```python
from build123d import *

# Parameters (mm, degrees)
SKETCH_3_W            = 95.96
SKETCH_3_H            = 56.19
EXTRUDE_2_DEPTH       = 2
SKETCH_4_W            = 97.56
SKETCH_4_H            = 57.79
SKETCH_4_W_2          = 95.96
SKETCH_4_H_2          = 56.19
CUT_EXTRUDE_1_DEPTH   = 2
SKETCH_5_R            = 3.6
SKETCH_5_R_2          = 2.4
EXTRUDE_1_DEPTH       = 4.6
EXTRUDE_START         = -2
EXTRUDE_3_DEPTH       = 2
CHAMFER_1_SIZE        = 1.8
SKETCH_8_W            = 10
SKETCH_8_H            = 75.2
EXTRUDE_3_2_DEPTH     = 2
FILLET_1_R            = 4
SKETCH_9_R            = 5.5
CUT_EXTRUDE_1_2_DEPTH = 2
SKETCH_11_R           = 2.4
SKETCH_11_R_2         = 1
EXTRUDE_4_DEPTH       = 4.6
SKETCH_14_W           = 10
SKETCH_14_H           = 1
EXTRUDE_4_2_DEPTH     = 3
CHAMFER_2_SIZE        = 3
CHAMFER_3_SIZE        = 3


with BuildPart() as part:
    # Эскиз3 → Бобышка-Вытянуть2 (new body)
    with BuildSketch(Plane.XY):
        with BuildLine():
            Line((-57.5, -37), (57.5, -37))
            ThreePointArc((57.5, -37), (59.267766953, -36.267766953), (60, -34.5))
            Line((60, -34.5), (60, 34.5))
            ThreePointArc((60, 34.5), (59.267766953, 36.267766953), (57.5, 37))
            Line((57.5, 37), (-57.5, 37))
            ThreePointArc((-57.5, 37), (-59.267766953, 36.267766953), (-60, 34.5))
            Line((-60, 34.5), (-60, -34.5))
            ThreePointArc((-60, -34.5), (-59.267766953, -36.267766953), (-57.5, -37))
        make_face()
        with Locations((0, 2.375)):
            Rectangle(SKETCH_3_W, SKETCH_3_H, mode=Mode.SUBTRACT)
    extrude(amount=EXTRUDE_2_DEPTH)

    # Эскиз4 → Cut-Extrude 1 (cut)
    with BuildSketch(Plane.XY.offset(2)):
        with Locations((0, 2.375)):
            Rectangle(SKETCH_4_W, SKETCH_4_H)
        with Locations((0, 2.375)):
            Rectangle(SKETCH_4_W_2, SKETCH_4_H_2, mode=Mode.SUBTRACT)
    extrude(amount=-CUT_EXTRUDE_1_DEPTH, mode=Mode.SUBTRACT)

    # Эскиз5 → Вытянуть-Тонкостенный1 (add)
    # profile 1 of 4: a face of its own
    with BuildSketch(Plane(origin=(0, 0, 0), x_dir=(-1, 0, 0), z_dir=(0, 0, -1))):
        with Locations((56.75, 33.75)):
            Circle(SKETCH_5_R)
        with Locations((56.75, 33.75)):
            Circle(SKETCH_5_R_2, mode=Mode.SUBTRACT)
    # profile 2 of 4: a face of its own
    with BuildSketch(Plane(origin=(0, 0, 0), x_dir=(-1, 0, 0), z_dir=(0, 0, -1))):
        with Locations((-56.75, 33.75)):
            Circle(SKETCH_5_R)
        with Locations((-56.75, 33.75)):
            Circle(SKETCH_5_R_2, mode=Mode.SUBTRACT)
    # profile 3 of 4: a face of its own
    with BuildSketch(Plane(origin=(0, 0, 0), x_dir=(-1, 0, 0), z_dir=(0, 0, -1))):
        with Locations((-56.75, -33.75)):
            Circle(SKETCH_5_R)
        with Locations((-56.75, -33.75)):
            Circle(SKETCH_5_R_2, mode=Mode.SUBTRACT)
    # profile 4 of 4: a face of its own
    with BuildSketch(Plane(origin=(0, 0, 0), x_dir=(-1, 0, 0), z_dir=(0, 0, -1))):
        with Locations((56.75, -33.75)):
            Circle(SKETCH_5_R)
        with Locations((56.75, -33.75)):
            Circle(SKETCH_5_R_2, mode=Mode.SUBTRACT)
    extrude(amount=EXTRUDE_1_DEPTH)

    # Эскиз7 → Extrude 3 (add)
    with BuildSketch(Plane.XY.offset(2).offset(EXTRUDE_START)):
        with BuildLine():
            Line((-60.6, 34.5), (-60.6, -34.5))
            ThreePointArc((-60.6, -34.5), (-59.692031022, -36.692031022), (-57.5, -37.6))
            Line((-57.5, -37.6), (57.5, -37.6))
            ThreePointArc((57.5, -37.6), (59.692031022, -36.692031022), (60.6, -34.5))
            Line((60.6, -34.5), (60.6, 34.5))
            ThreePointArc((60.6, 34.5), (59.692031022, 36.692031022), (57.5, 37.6))
            Line((57.5, 37.6), (-57.5, 37.6))
            ThreePointArc((-57.5, 37.6), (-59.692031022, 36.692031022), (-60.6, 34.5))
        make_face()
        with BuildLine():
            Line((-60, 34.5), (-60, -34.5))
            ThreePointArc((-60, -34.5), (-59.267766953, -36.267766953), (-57.5, -37))
            Line((-57.5, -37), (57.5, -37))
            ThreePointArc((57.5, -37), (59.267766953, -36.267766953), (60, -34.5))
            Line((60, -34.5), (60, 34.5))
            ThreePointArc((60, 34.5), (59.267766953, 36.267766953), (57.5, 37))
            Line((57.5, 37), (-57.5, 37))
            ThreePointArc((-57.5, 37), (-59.267766953, 36.267766953), (-60, 34.5))
        make_face(mode=Mode.SUBTRACT)
    extrude(amount=EXTRUDE_3_DEPTH)

    # Фаска1
    chamfer_1_edges = [part.edges().sort_by_distance(p)[0] for p in [
        (0, 31.27, 2),
        (-48.78, 2.375, 2),
        (0, -26.52, 2),
        (48.78, 2.375, 2),
    ]]
    chamfer(chamfer_1_edges, length=CHAMFER_1_SIZE)

    # Эскиз8 → Extrude 3 2 (add)
    with BuildSketch(Plane.XY.offset(2)):
        with Locations((62.5, 0)):
            Rectangle(SKETCH_8_W, SKETCH_8_H)
        with Locations((-62.5, 0)):
            Rectangle(SKETCH_8_W, SKETCH_8_H)
    extrude(amount=-EXTRUDE_3_2_DEPTH)

    # Скругление1
    fillet_1_edges = [part.edges().sort_by_distance(p)[0] for p in [
        (67.5, 37.6, 1),
        (67.5, -37.6, 1),
        (-67.5, -37.6, 1),
        (-67.5, 37.6, 1),
    ]]
    fillet(fillet_1_edges, radius=FILLET_1_R)

    # Эскиз9 → Cut-Extrude 1 2 (cut)
    with BuildSketch(Plane.XY.offset(2)):
        with Locations((59.1, 9.48)):
            Circle(SKETCH_9_R)
        with Locations((59.1, -6.52)):
            Circle(SKETCH_9_R)
    extrude(amount=-CUT_EXTRUDE_1_2_DEPTH, mode=Mode.SUBTRACT)

    # Эскиз11 → Extrude 4 (add)
    # profile 1 of 4: a face of its own
    with BuildSketch(Plane(origin=(0, 0, 0), x_dir=(-1, 0, 0), z_dir=(0, 0, -1))):
        with Locations((-56.75, 33.75)):
            Circle(SKETCH_11_R)
        with Locations((-56.75, 33.75)):
            Circle(SKETCH_11_R_2, mode=Mode.SUBTRACT)
    # profile 2 of 4: a face of its own
    with BuildSketch(Plane(origin=(0, 0, 0), x_dir=(-1, 0, 0), z_dir=(0, 0, -1))):
        with Locations((56.75, 33.75)):
            Circle(SKETCH_11_R)
        with Locations((56.75, 33.75)):
            Circle(SKETCH_11_R_2, mode=Mode.SUBTRACT)
    # profile 3 of 4: a face of its own
    with BuildSketch(Plane(origin=(0, 0, 0), x_dir=(-1, 0, 0), z_dir=(0, 0, -1))):
        with Locations((56.75, -33.75)):
            Circle(SKETCH_11_R)
        with Locations((56.75, -33.75)):
            Circle(SKETCH_11_R_2, mode=Mode.SUBTRACT)
    # profile 4 of 4: a face of its own
    with BuildSketch(Plane(origin=(0, 0, 0), x_dir=(-1, 0, 0), z_dir=(0, 0, -1))):
        with Locations((-56.75, -33.75)):
            Circle(SKETCH_11_R)
        with Locations((-56.75, -33.75)):
            Circle(SKETCH_11_R_2, mode=Mode.SUBTRACT)
    extrude(amount=EXTRUDE_4_DEPTH)

    # Эскиз14 → Extrude 4 2 (add)
    with BuildSketch(Plane(origin=(0, 0, 0), x_dir=(-1, 0, 0), z_dir=(0, 0, -1))):
        with Locations((-59.1, 17.98)):
            Rectangle(SKETCH_14_W, SKETCH_14_H)
        with Locations((-59.1, 1.58)):
            Rectangle(SKETCH_14_W, SKETCH_14_H)
        with Locations((-59.1, -16.02)):
            Rectangle(SKETCH_14_W, SKETCH_14_H)
    extrude(amount=EXTRUDE_4_2_DEPTH)

    # Фаска2
    chamfer_2_edges = [part.edges().sort_by_distance(p)[0] for p in [
        (59.1, 18.48, 0),
    ]]
    chamfer(chamfer_2_edges, length=CHAMFER_2_SIZE - 0.0001)  # a hair under: the kernel refuses the full size

    # Фаска3
    chamfer_3_edges = [part.edges().sort_by_distance(p)[0] for p in [
        (59.1, -16.52, 0),
    ]]
    chamfer(chamfer_3_edges, length=CHAMFER_3_SIZE - 0.0001)  # a hair under: the kernel refuses the full size


solid = part.part
```
Source: CAD feature listing. Evaluate the final solid. Frame: model axes, mm. A direction names the side the tool comes from. Round coordinates to 2 decimals unless told otherwise and drop trailing zeros. Loops run counter-clockwise (first coordinate to the right, second up) from the corner with the lowest first, then second, coordinate; pieces in that order, holes last. Notation, with made-up numbers: M 78.25,65.25 L 114.25,65.25 A19 ccw 114.25,83.25 Z; hole C 4,75 d8. An arc over 180 degrees is marked long. Use a Markdown table: item, result. Add a question column.
1. Ray query, line 1 along Y through (x, z) = (59.1, 1.5); line 2 along X through (y, z) = (34, -3); line 3 along Y through (x, z) = (-56.75, -1.2). Return the intervals inside material, ascending. Write a range as [from, to].
2. Set-up query: faces 4 (the flat face through (64.1, -17, -1)), 5 (the flat face through (59, 17.48, -1)), 6 (the flat face through (54.1, -17, -1)), 7 (the cylindrical face through (53.316, -32.669, -2.268)). Return all of +Z, -Z, +X, -X, +Y, -Y with unobstructed straight access to the full face (end or side cutting, diameter ignored); none if empty.
3. Pull-direction query (Y, two-part tool) for faces 1 (the flat face through (64.1, 19, -1)), 2 (the cylindrical face through (-66.297, -36.459, 0.986)), 3 (the flat face through (59, 2.08, -1)); classes: +Y half, -Y half, draft (parallel to the pull), parting line (faces both ways), or undercut.
4. Cut plane B-B, the plane y = 9.48. Output: boundary loops of the cut face in (x, z).
5. Cut plane D-D, the plane y = 25. Output: boundary loops of the cut face in (x, z), and give its area (3 significant figures).
6. Cut plane A-A, the plane x = -30. Output: boundary loops of the cut face in (y, z), and give its area (3 significant figures).
7. Cut plane C-C, the plane z = -1.5. State how many separate pieces and enclosed holes the cut face has, and give its area (3 significant figures).
8. Contact query for flat-ended pins moving along their axis: pin 1 (1.1 mm diameter, centred on x = 59.5, y = 1.5, fed in from -Z); pin 2 (0.5 mm diameter, centred on y = 1.5, z = -1, fed in from +X); pin 3 (1.5 mm diameter, centred on x = 60, z = -1.5, fed in from +Y). Output: stop coordinate, or through.
Solution:
| question | item | result |
|---|---|---|
| 1 | line 1 | y = [-37.6, -12.02], [-1.02, 3.98], [14.98, 37.6] |
| 1 | line 2 | x = [-60.34, -57.72], [-55.78, -53.16], [53.16, 55.78], [57.72, 60.34] |
| 1 | line 3 | y = [-37.35, -34.75], [-32.75, -30.15], [30.15, 32.75], [34.75, 37.35] |
| 2 | face 4 | -Z, +X, +Y, -Y |
| 2 | face 5 | -Z, +X, -X |
| 2 | face 6 | -Z, -X |
| 2 | face 7 | -Z |
| 3 | face 1 | draft |
| 3 | face 2 | -Y half |
| 3 | face 3 | undercut |
| 4 | outline | M -67.5,0 L -48.78,0 L -48.78,0.2 L -50.58,2 L -67.5,2 Z; M 48.78,0 L 53.6,0 L 53.6,2 L 50.58,2 L 48.78,0.2 Z; M 64.6,0 L 67.5,0 L 67.5,2 L 64.6,2 Z |
| 5 | outline | M -67.5,0 L -48.78,0 L -48.78,0.2 L -50.58,2 L -67.5,2 Z; M 48.78,0 L 67.5,0 L 67.5,2 L 50.58,2 L 48.78,0.2 Z |
| 5 | area | 71.6 mm2 |
| 6 | outline | M -37.6,0 L -26.52,0 L -26.52,0.2 L -28.32,2 L -37.6,2 Z; M 31.27,0 L 37.6,0 L 37.6,2 L 33.07,2 L 31.27,0.2 Z |
| 6 | area | 31.6 mm2 |
| 7 | separate pieces | 7 |
| 7 | enclosed holes | 4 |
| 7 | area | 210 mm2 |
| 8 | pin 1 | stops at z = -3 |
| 8 | pin 2 | stops at x = 64.1 |
| 8 | pin 3 | stops at y = 36.34 |
